Here's how the part is built. I have some questions about the finished solid (model axes, mm). A direction names the side the tool comes from. Coordinates: 2 decimals unless noted, no trailing zeros. Order: outer loops, then holes, each group sorted by start corner. A loop starts at its lowest first (then second) coordinate and runs counter-clockwise, first axis right, second up. Notation, with made-up numbers: (84, 30) - (143, 30) arc R24 ccw to (143, 43) - close; hole circle Ø3 at (-16.5, 68.25). An arc over 180 degrees is marked (long way). Answer as CSV lines item,"result". Start each with the question number.
Q1. For faces 1 (the face through (20.9, -0.9, 7)), 2 (the face through (0, -1, 39)), which set-ups out of +Z, -Z, +X, -X, +Y, -Y let a thin tool reach every point of the face, with its end or its side?
Q2. I need wall thicknesses on line 1 (Z direction, x = 8.5, y = 40.5); line 2 (X direction, y = -43, z = 17); line 3 (Z direction, x = 25.5, y = -57.5). Which ranges of each line are inside material? Lowest first, please.
Q3. Suppose I cut it at D-D (x = 29). Please give me the cut outline in (y, z), then the cut area to 3 significant figures.
Q4. Suppose I cut it at C-C (z = 26.5). Please give me the cut outline in (x, y), then the cut area to 3 significant figures.
Q5. Suppose I cut it at A-A (y = 15.5). Please give me the cut outline in (x, z).
Q6. Suppose I cut it at B-B (x = 17). Please give me the cut outline in (y, z).
Q7. Thinking about a two-plate mould opening in Z: for faces 3 (the face through (16, -1, 0)), 4 (the face through (35.56, -0.89, 2.48)), 5 (the face through (3, -63.5, 35)), 6 (the face through (17, -1, 76.2)), which applies, released by +Z, released by -Z, zero draft, split by the parting line, or undercut?
from build123d import *

# Parameters (mm, degrees)
F1_DEPTH = 63.5


with BuildPart() as f1:
    # F0 (on Front) → F1 (new body, symmetric)
    with BuildSketch(Plane.XZ):
        with BuildLine():
            Line((0, 76.2), (0, 0))
            Line((0, 0), (33.02, 0))
            ThreePointArc((33.02, 0), (35.56, 2.54), (33.02, 5.08))
            Line((33.02, 5.08), (8.410474, 8.977766))
            ThreePointArc((8.410474, 8.977766), (5.480366, 10.618705), (4.318, 13.769437))
            Line((4.318, 13.769437), (4.318, 62.398901))
            ThreePointArc((4.318, 62.398901), (5.480366, 65.549634), (8.410474, 67.190573))
            Line((8.410474, 67.190573), (33.417344, 71.151272))
            ThreePointArc((33.417344, 71.151272), (35.55217, 73.859286), (33.02, 76.2))
            Line((33.02, 76.2), (0, 76.2))
        make_face()
    extrude(amount=F1_DEPTH, both=True)


solid = f1.part
Here are the results:
1,face 1,"+X, +Y, -Y"
1,face 2,"+Z, -Z, -X, +Y, -Y"
2,line 1,"z = 0 to 8.96, 67.2 to 76.2"
2,line 2,"x = 0 to 4.32"
2,line 3,"z = 0 to 6.27, 69.9 to 76.2"
3,outline,"(-63.5, 0) - (63.5, 0) - (63.5, 5.72) - (-63.5, 5.72) - close; (-63.5, 70.45) - (63.5, 70.45) - (63.5, 76.2) - (-63.5, 76.2) - close"
3,area,"1,460 mm²"
4,outline,"(0, -63.5) - (4.32, -63.5) - (4.32, 63.5) - (0, 63.5) - close"
4,area,"548 mm²"
5,outline,"(0, 0) - (33.02, 0) arc R2.54 ccw to (33.02, 5.08) - (8.41, 8.98) arc R4.85 cw to (4.32, 13.77) - (4.32, 62.4) arc R4.85 cw to (8.41, 67.19) - (33.42, 71.15) arc R2.54 ccw to (33.02, 76.2) - (0, 76.2) - close"
6,outline,"(-63.5, 0) - (63.5, 0) - (63.5, 7.62) - (-63.5, 7.62) - close; (-63.5, 68.55) - (63.5, 68.55) - (63.5, 76.2) - (-63.5, 76.2) - close"
7,face 3,"released by -Z"
7,face 4,"undercut"
7,face 5,"zero draft"
7,face 6,"released by +Z"
